CAD build for the part. Positions are in the model's coordinates, mm. A direction names the side the tool comes from. Give positions to 0.01 mm unless a question says otherwise; leave off trailing zeros. Order: outer loops, then holes, each group sorted by start corner. A loop starts at its lowest first (then second) coordinate and runs counter-clockwise, first axis right, second up. Notation, with made-up numbers: (65.5, 1) -> (74.5, 1) arc R11 cw to (74.5, 15) -> close; hole circle Ø5 at (71, -16). An arc over 180 degrees is marked (long way). Use one line per item in the form item = value. Start each with the question number.
1) Probe line 1 (X direction, y = 3.45, z = -46.5) (3 decimals); line 2 (X direction, y = 0.4, z = 77); line 3 (Z direction, x = -46, y = 0.8). List the from-to ranges inside material, lowest first.
2) Drop flat-ended pins along their axis: P1, Ø1.4, axis at y = 3, z = 91.5, coming from the -X side; P2, Ø1.4, axis at x = 41, y = 2.5, coming from the +Z side; P3, Ø1.4, axis at x = -38, y = 2, coming from the -Z side. Give the stop position or say it passes through.
3) Tool access for faces 5 (the face through (38, 2, 88.9)), 6 (the face through (-19.05, 2, 1)), 7 (the face through (-38, 2, 93.663)), 8 (the face through (-44.293, 2, 91)), 9 (the face through (6.35, 2, 91)): list every direction of +Z, -Z, +X, -X, +Y, -Y with a clear straight run to the whole face (end or side of a thin tool).
4) Mould opens along Z. For faces 1 (the face through (-27.305, 2, 1)), 2 (the face through (38, 2, -93.663)), 3 (the face through (41, 2, -82.55)), 4 (the face through (-6.35, 2, -91)) say: pulls with the +Z half, pulls with the -Z half, needs draft (parallel to the pull), parting line crosses it, or undercut.
5) Cut at B-B, the plane z = -56. State how many separate pieces and enclosed holes the cut face has, and give its area (3 significant figures).
6) Cut at A-A, the plane x = 10. Give the cut face in (y, z), and give its area (3 significant figures).
from build123d import *

# Parameters (mm, degrees)
SKETCH1_W           = 114.3
SKETCH1_H           = 177.8
SKETCH1_W_2         = 101.6
SKETCH1_H_2         = 165.1
BOSS_EXTRUDE1_DEPTH = 4.7625
SKETCH2_W           = 12.38677804
SKETCH2_H           = 4.7625
SKETCH2_W_2         = 12.7
BOSS_EXTRUDE2_DEPTH = 4.7625
SKETCH3_W           = 12.7
SKETCH3_H           = 4.7625
BOSS_EXTRUDE3_DEPTH = 4.7625
FILLET1_R           = 2.54
SKETCH7_W           = 12.7
SKETCH7_H           = 165.1
SKETCH7_W_2         = 3.81
SKETCH7_H_2         = 152.4
BOSS_EXTRUDE6_DEPTH = 4.7625
FILLET3_R           = 2.54
FILLET4_R           = 1.905


with BuildPart() as part:
    # Sketch1 → Boss-Extrude1 (new body)
    with BuildSketch(Plane(origin=(0, 0, 0), x_dir=(1, 0, 0), z_dir=(0, 1, 0))):
        Rectangle(SKETCH1_W, SKETCH1_H)
        Rectangle(SKETCH1_W_2, SKETCH1_H_2, mode=Mode.SUBTRACT)
    extrude(amount=BOSS_EXTRUDE1_DEPTH)

    # Sketch2 → Boss-Extrude2 (add)
    with BuildSketch(Plane.XY.offset(88.9)):
        with Locations((-38.1, 2.38125)):
            Rectangle(SKETCH2_W, SKETCH2_H)
        with Locations((12.7, 2.38125)):
            Rectangle(SKETCH2_W_2, SKETCH2_H)
    extrude(amount=BOSS_EXTRUDE2_DEPTH)

    # Sketch3 → Boss-Extrude3 (add)
    with BuildSketch(Plane(origin=(0, 0, -88.9), x_dir=(-1, 0, 0), z_dir=(0, 0, -1))):
        with Locations((-38.1, 2.38125)):
            Rectangle(SKETCH3_W, SKETCH3_H)
        with Locations((12.7, 2.38125)):
            Rectangle(SKETCH3_W, SKETCH3_H)
    extrude(amount=BOSS_EXTRUDE3_DEPTH)

    # Fillet1
    fillet1_edges = [part.edges().sort_by_distance(p)[0] for p in [
        (50.8, 2.38125, 82.55),
        (50.8, 2.38125, -82.55),
        (-50.8, 2.38125, -82.55),
        (-50.8, 2.38125, 82.55),
    ]]
    fillet(fillet1_edges, radius=FILLET1_R)

    # Sketch7 → Boss-Extrude6 (add)
    # profile 1 of 2: a face of its own
    with BuildSketch(Plane(origin=(0, 4.7625, 0), x_dir=(1, 0, 0), z_dir=(0, 1, 0))):
        with Locations((-25.4, 0)):
            Rectangle(SKETCH7_W, SKETCH7_H)
        with Locations((-25.4, 0)):
            Rectangle(SKETCH7_W_2, SKETCH7_H_2, mode=Mode.SUBTRACT)
    # profile 2 of 2: a face of its own
    with BuildSketch(Plane(origin=(0, 4.7625, 0), x_dir=(1, 0, 0), z_dir=(0, 1, 0))):
        with Locations((25.4, 0)):
            Rectangle(SKETCH7_W, SKETCH7_H)
        with Locations((25.4, 0)):
            Rectangle(SKETCH7_W_2, SKETCH7_H_2, mode=Mode.SUBTRACT)
    extrude(amount=-BOSS_EXTRUDE6_DEPTH)

    # Fillet3
    fillet3_edges = [part.edges().sort_by_distance(p)[0] for p in [
        (-31.75, 2.38125, 82.55),
        (-31.75, 2.38125, -82.55),
        (-19.05, 2.38125, -82.55),
        (-19.05, 2.38125, 82.55),
        (19.05, 2.38125, 82.55),
        (19.05, 2.38125, -82.55),
        (31.75, 2.38125, -82.55),
        (31.75, 2.38125, 82.55),
    ]]
    fillet(fillet3_edges, radius=FILLET3_R)

    # Fillet4
    fillet4_edges = [part.edges().sort_by_distance(p)[0] for p in [
        (27.305, 2.38125, -76.2),
        (23.495, 2.38125, -76.2),
        (27.305, 2.38125, 76.2),
        (23.495, 2.38125, 76.2),
        (-23.495, 2.38125, 76.2),
        (-27.305, 2.38125, 76.2),
        (-23.495, 2.38125, -76.2),
        (-27.305, 2.38125, -76.2),
    ]]
    fillet(fillet4_edges, radius=FILLET4_R - 0.0001)  # a hair under: the kernel refuses the full size


solid = part.part
Result:
q1.line_1 = -57.15 to -50.8, -31.75 to -27.305, -23.495 to -19.05, 19.05 to 23.495, 27.305 to 31.75, 50.8 to 57.15
q1.line_2 = -57.15 to -50.8, -31.75 to -19.05, 19.05 to 31.75, 50.8 to 57.15
q1.line_3 = -88.9 to -82.55, 82.55 to 88.9
q2.P1 = -44.29
q2.P2 = 88.9
q2.P3 = -88.9
q3.face_5 = +Z, +X, +Y, -Y
q3.face_6 = +Y, -Y
q3.face_7 = +Z, +X, -X, +Y, -Y
q3.face_8 = +Z, -X, +Y, -Y
q3.face_9 = +Z, +Y, -Y
q4.face_1 = undercut
q4.face_2 = pulls with the -Z half
q4.face_3 = undercut
q4.face_4 = needs draft
q5.separate_pieces = 6
q5.enclosed_holes = 0
q5.area = 145 mm²
q6.outline = (0, -88.9) -> (4.76, -88.9) -> (4.76, -82.55) -> (0, -82.55) -> close; (0, 82.55) -> (4.76, 82.55) -> (4.76, 93.66) -> (0, 93.66) -> close
q6.area = 83.2 mm²
